Can you work these out from the model? Positions are in its coordinate system, mm. A direction names the side the tool comes from. Coordinates: 2 decimals unless noted, no trailing zeros. Write each loop counter-clockwise with the first axis right and the second up, starting at its lowest first coordinate (ties: lowest second). Pieces come first, ordered by that corner, then holes. Notation, with made-up numbers: (-37.5, 14) -> (4.5, 14) arc R31 cw to (4.5, 52) -> close; hole circle Ø8 at (30.25, 56). An arc over 180 degrees is marked (long way). Use one line per item in the form item = value.
Autodesk Inventor part; units mm, degrees
ref_plane "YZ Plane" through (0, 0, 0) normal (1, 0, 0) x (0, 1, 0)
ref_plane "XZ Plane" through (0, 0, 0) normal (0, 1, 0) x (-1, 0, 0)
ref_plane "XY Plane" through (0, 0, 0) normal (0, 0, 1) x (1, 0, 0)
sketch "Sketch1" plane through (0, 0, 0) normal (0, 1, 0) x (-1, 0, 0)
  arc A0 (6, -2.425) -> (6, -5.575) centre (6, -4) ccw construction
  line L0 (6, -2.425) -> (8, -2.425) construction
  arc A1 (8, -5.575) -> (8, -2.425) centre (8, -4) ccw construction
  line L1 (8, -5.575) -> (6, -5.575) construction
  arc A2 (6, -18.425) -> (6, -21.575) centre (6, -20) ccw construction
  line L2 (6, -18.425) -> (8, -18.425) construction
  arc A3 (8, -21.575) -> (8, -18.425) centre (8, -20) ccw construction
  line L3 (8, -21.575) -> (6, -21.575) construction
  line L4 (18, 0) -> (18, -4)
  line L5 (2, 0) -> (18, 0)
  line L6 (2, -24) -> (2, 0)
  line L7 (18, -24) -> (2, -24)
  line L8 (18, -20) -> (18, -24)
  arc A4 (18, -6) -> (18, -18) centre (18, -12) ccw
  line L9 (18, -6) -> (18, -4)
  line L10 (18, -20) -> (18, -18)
  arc A5 (18, -4) -> (18, -20) centre (18, -12) ccw
  circle A6 centre (8, -20) radius 2.375
  circle A7 centre (8, -4) radius 2.375
  point P0 (0, 0)
  point P1 (0, 0)
  dimension "d0" = 16
  dimension "d2" = 8
  dimension "d4" = 6
  dimension "d5" = 1.575
  dimension "d6" = 2
  dimension "d7" = 1.575
  dimension "d8" = 2
  dimension "d11" = 4.75
  dimension "d12" = 4.75
extrude "Extrusion1" add sketch "Sketch1" along normal blind 8 contours L4 A5 L8 L7 L6 L5
extrude "Extrusion3" add sketch "Sketch1" along normal blind 3 contours A6 | A7
sketch "Sketch2" plane through (-8, 3, -4) normal (0, 1, 0) x (1, 0, 0)
  circle A0 centre (0, 0) radius 2.375
  circle A1 centre (0, 16) radius 2.375
  circle A2 centre (0, 0) radius 2.375
  circle A3 centre (0, 0) radius 1.575
  circle A4 centre (0, 16) radius 1.575
  point P0 (8, -4)
  dimension "d19" = 3.15
  dimension "d20" = 3.15
extrude "Extrusion4" cut sketch "Sketch2" against normal through all contours A3 | A4
extrude "Extrusion2" [suppressed]
sketch "Sketch3" plane through (-18, 0, 0) normal (0, 0, 1) x (1, 0, 0)
  line L0 (0, 0) -> (16, 0)
  line L1 (16, 0) -> (16, 8)
  line L2 (0, 8) -> (16, 8)
  line L3 (0, 0) -> (0, 8)
  line L4 (8.425, 3) -> (8.425, 0)
  line L5 (16, 0) -> (0, 0)
  line L6 (0, 0) -> (0, 8)
  line L7 (16, 8) -> (0, 8)
  line L8 (16, 0) -> (16, 8)
  point P0 (18, 0)
sketch "Sketch4" plane through (-2, 0, -24) normal (0, 0, -1) x (-1, 0, 0)
  line L0 (0, 0) -> (16, 0)
  line L1 (16, 0) -> (16, 8)
  line L2 (0, 8) -> (16, 8)
  line L3 (0, 0) -> (0, 8)
  point P0 (-2, 0)
extrude "Extrusion6" cut sketch "Sketch3" against normal blind 0.25
extrude "Extrusion7" cut sketch "Sketch4" against normal blind 0.25
sketch "Sketch5" plane through (-2, 0, -0.25) normal (1, 0, 0) x (0, 0, -1)
  line L0 (23.5, 0) -> (23.5, 8)
  line L1 (0, 8) -> (23.5, 8)
  line L2 (0, 8) -> (0, 0)
  line L3 (0, 0) -> (23.5, 0)
  point P0 (-0.25, 0)
extrude "Extrusion8" cut sketch "Sketch5" against normal blind 2
chamfer "Chamfer1" [suppressed]
chamfer "Chamfer2" [suppressed]
sketch "Sketch11" plane through (-2, 0, -23.75) normal (0, 0, -1) x (-1, 0, 0)
  line L0 (2, 8) -> (2, 0)
  line L1 (16, 0) -> (2, 0)
  line L2 (16, 8) -> (16, 0)
  line L3 (2, 8) -> (16, 8)
  line L4 (2, 0) -> (16, 0)
  line L5 (16, 0) -> (2, 1.2248)
  line L6 (2, 0) -> (2, 8)
  line L7 (16, 0) -> (30.0535, 0) construction
  point P0 (-2, 0)
  dimension "d46" = 175
extrude "Extrusion11" cut sketch "Sketch11" against normal through all contours L5 L1 L0
sketch "Sketch12" plane through (-2, 0, -23.75) normal (0, 0, -1) x (-1, 0, 0)
  line L0 (2, 1.2248) -> (16, 0)
  line L1 (16, 8) -> (16, 0)
  line L2 (2, 8) -> (16, 8)
  line L3 (2, 8) -> (2, 1.2248)
  line L4 (16, 0) -> (2, 1.2248)
  line L5 (2, 1.2248) -> (2, 8)
  line L6 (16, 8) -> (2, 8)
  line L7 (16, 0) -> (16, 8)
  point P0 (-2, 0)
extrude "Extrusion12" cut sketch "Sketch12" against normal blind 0.5
sketch "Sketch13" plane through (-18, 0, -0.25) normal (0, 0, 1) x (1, 0, 0)
  line L0 (0, 0) -> (14, 1.2248)
  line L1 (14, 1.2248) -> (14, 8)
  line L2 (0, 8) -> (14, 8)
  line L3 (0, 0) -> (0, 8)
  point P0 (18, 0)
extrude "Extrusion13" cut sketch "Sketch13" against normal blind 0.5
sketch "Sketch15" plane through (0, 8, 0) normal (0, 1, 0) x (1, 0, 0)
  arc A0 (-18, 4) -> (-18, 20) centre (-18, 12) ccw
  arc A1 (-18, 6) -> (-18, 18) centre (-18, 12) ccw
  line L0 (-18, 18) -> (-18, 20)
  line L1 (-18, 4) -> (-18, 0.75)
  line L2 (-18, 6) -> (-18, 4)
  point P0 (0, 0)
  dimension "d53" = 12
extrude "Extrusion14" add sketch "Sketch15" against normal blind 8
sketch "Sketch16" plane through (0, 8, 0) normal (0, 1, 0) x (1, 0, 0)
  arc A0 (-18, 4) -> (-18, 20) centre (-18, 12) ccw
  arc A1 (-18, 6) -> (-18, 18) centre (-18, 12) ccw
  line L0 (-18, 0.75) -> (-18, 6)
  line L1 (-18, 23.25) -> (-18, 18)
  point P0 (0, 0)
extrude "Extrusion15" cut sketch "Sketch16" against normal blind 2
chamfer "Chamfer3" distance 2 angle 45 2 edges at (-18, 3, -6) (-18, 3, -18)
equation "\"d12\" = d11"
properties part number "hotend_holder_clamp" material "ABS Plastic"
Q1. Suppose I cut it at D-D (x = -15.5). Write out the boundary of the cut face in (y, z).
Return value:
outline = (0, -19.6) -> (0.22, -19.6) -> (0.22, -23.25) -> (8, -23.25) -> (8, -19.6) -> (6, -19.6) -> (6, -17.45) -> (0, -17.45) -> close; (0, -6.55) -> (6, -6.55) -> (6, -4.4) -> (8, -4.4) -> (8, -0.75) -> (0.22, -0.75) -> (0.22, -4.4) -> (0, -4.4) -> close
Q2. Thinking about a two-plate mould opening in Z: for faces 1 (the flat face through (-11, 4, -23.25)), 2 (the cylindrical face through (-9.573, 1.883, -20.069)), 3 (the flat face through (-9.5, 8, -12.2)), 4 (the cylindrical face through (-7.49, 5.46, -1.68)), which applies, released by +Z, released by -Z, zero draft, split by the parting line, or undercut?
Return value:
face_1 = released by -Z
face_2 = undercut
face_3 = zero draft
face_4 = undercut
Q3. Suppose I cut it at C-C (z = -12). Write out the boundary of the cut face in (x, y), then the cut area to 3 significant figures.
Return value:
outline = (-12, 0) -> (-10, 0) -> (-10, 0.7) -> (-4, 1.22) -> (-4, 8) -> (-10, 8) -> (-10, 6) -> (-12, 6) -> close
area = 54.2 mm2
Q4. If I drill on line 1 (Z direction, x = -8, y = 5.5) (3 decimals); line 2 (Z direction, x = -8, y = 1.9) (3 decimals); line 3 (X direction, y = 1.5, z = -4) (3 decimals), over which ranges is the centre line in solid material (lowest first)? Write a range as from..to.
Return value:
line_1 = -23.25..-22.375, -17.625..-6.375, -1.625..-0.75
line_2 = -23.25..-21.575, -18.425..-5.575, -2.425..-0.75
line_3 = -18..-9.575, -6.425..-4
Q5. For faces 5 (the flat face through (-9.54, 0.74, -12.16)), 6 (the cylindrical face through (-10, 7, -12)), 7 (the flat face through (-10, 3, -4)), 8 (the flat face through (-17, 3.042, -5.183)), which set-ups out of +Z, -Z, +X, -X, +Y, -Y let a thin tool reach every point of the face, with its end or its side?
Return value:
face_5 = +X, -Y
face_6 = -X, +Y
face_7 = +Y
face_8 = -X, +Y, -Y
Q6. Suppose I cut it at A-A (x = -8). Write out the boundary of the cut face in (y, z) (3 decimals), then the cut area to 3 significant figures.
Return value:
outline = (0.875, -23.25) -> (8, -23.25) -> (8, -22.375) -> (3, -22.375) -> (3, -21.575) -> (0.875, -21.575) -> close; (0.875, -18.425) -> (3, -18.425) -> (3, -17.625) -> (8, -17.625) -> (8, -6.375) -> (3, -6.375) -> (3, -5.575) -> (0.875, -5.575) -> close; (0.875, -2.425) -> (3, -2.425) -> (3, -1.625) -> (8, -1.625) -> (8, -0.75) -> (0.875, -0.75) -> close
area = 99.4 mm2
Q7. Suppose I cut it at B-B (y = 5.5). Write out the boundary of the cut face in (x, z) (3 decimals).
Return value:
outline = (-18, -23.25) -> (-4, -23.25) -> (-4, -0.75) -> (-18, -0.75) -> (-18, -4) -> (-16.028, -6.333) arc R6 cw to (-16.028, -17.667) -> (-18, -20) -> close; hole circle Ø4.75 at (-8, -20); hole circle Ø4.75 at (-8, -4)
Q8. Will these pins go through, and if not, where does the flat tip stop? pin 1 (3.5 mm diameter, centred on x = -8, z = -20, fed in from +Y); pin 2 (2.5 mm diameter, centred on x = -14, z = -14.5, fed in from +Y).
Return value:
pin_1 = 3
pin_2 = through
